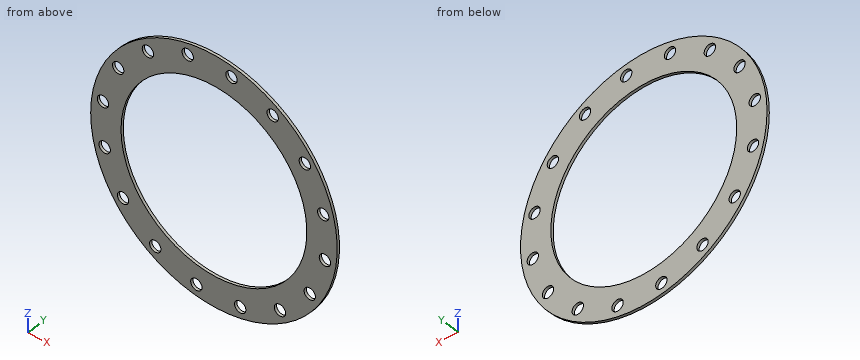
Autodesk Inventor part; units mm, degrees
ref_plane "YZ Plane" through (0, 0, 0) normal (1, 0, 0) x (0, 1, 0)
ref_plane "XZ Plane" through (0, 0, 0) normal (0, 1, 0) x (-1, 0, 0)
ref_plane "XY Plane" through (0, 0, 0) normal (0, 0, 1) x (1, 0, 0)
sketch "Sketch1" plane through (0, 0, 0) normal (0, 1, 0) x (-1, 0, 0)
  circle A0 centre (0, 0) radius 213
  circle A1 centre (0, 0) radius 282.5
  line L0 (282.5, 0) -> (213, 0)
  line L1 (-213, 0) -> (-282.5, 0)
  line L2 (0, 213) -> (0, 282.5)
  point P0 (247.75, 0)
  point P1 (-247.75, 0)
  point P2 (0, 247.75)
  dimension "d1" = 565
  dimension "d4" = 426
extrude "Extrusion1" add sketch "Sketch1" along normal blind 6 contours L0 A1 L1 A0 | A0 L2 A1 L0 | A0 L1 A1 L2
sketch "Sketch2" plane through (0, 0, 0) normal (0, -1, 0) x (1, 0, 0)
  circle A0 centre (0, 0) radius 282.5
  circle A1 centre (0, 0) radius 213
  circle A2 centre (40.2819, 254.3297) radius 13
  circle A3 centre (0, 0) radius 213
  line L0 (40.2819, 254.3297) -> (0, 0)
  point P0 (0, 213)
  point P1 (265, 0)
  dimension "d5" = 257.5
  dimension "d7" = 26
extrude "Cut1" cut sketch "Sketch2" against normal blind 6 contours A2
pattern_circular "Circular Pattern1" count 16 over 360 about axis through (0, 0, 0) along (0, 1, 0) of "Cut1"
equation "\"d1\" = Charging_hatch_width"
equation "\"d4\" = Accsess_hatch_diameter"
equation "\"d9\" = Thickness"
equation "\"BendRadius\" = Thickness"
equation "\"BendReliefWidth\" = Thickness"
equation "\"BendReliefDepth\" = 0.5 * Thickness"
equation "\"CornerReliefSize\" = 4 * Thickness"
equation "\"MinimumRemnant\" = 2 * Thickness"
equation "\"TransitionRadius\" = BendRadius"
equation "\"JacobiRadiusSize\" = BendRadius"
equation "\"GapSize\" = Thickness"
equation "\"d8\" = Thickness"
properties part number "TZS 1203 accses hatch flange" material "Steel"
Build history of the part. All positions in model axes, mm. Round coordinates to 2 decimals unless told otherwise and drop trailing zeros. Loops run counter-clockwise (first coordinate to the right, second up) from the corner with the lowest first, then second, coordinate; pieces in that order, holes last. Notation, with made-up numbers: M 58,53.5 L 75,53.5 A19 cw 75,89.5 Z; hole C 1,82 d10. An arc over 180 degrees is marked long. Answer as CSV lines item,"result".
1. Cut at A-A on x = 0. Write the cut outline in (y, z).
Resolved:
outline,"M 0,-282.5 L 6,-282.5 L 6,-213 L 0,-213 Z; M 0,213 L 6,213 L 6,282.5 L 0,282.5 Z"
2. Flat gauge pins, fed straight in: P1, Ø1.5, axis at y = 1, z = 131.5, coming from the -X side; P2, Ø6, axis at x = 52, z = 213.5, coming from the -Y side; P3, Ø3, axis at x = 192, y = 0.5, coming from the -Z side; P4, Ø3, axis at x = 223, y = 2.5, coming from the -Z side. Where does each tip first touch, or does it go through?
Resolved:
P1,"stops at x = -250.42"
P2,"stops at y = 0"
P3,"stops at z = -208.6"
P4,"stops at z = -175.34"
3. Wall check: probe 1 along X at (y, z) = (4.15, 150.5); probe 2 along X at (y, z) = (4.6, -256.5); probe 3 along Z at (x, y) = (-146, 3.45). Give the ranges that are in metal, low to high. Write a range as [from, to].
Resolved:
probe 1,"x = [-239.07, -150.73], [150.73, 195.35], [221.29, 239.07]"
probe 2,"x = [-118.38, -53.1], [-27.46, 48.64], [71.58, 118.38]"
probe 3,"z = [-241.85, -225.7], [-213.41, -155.09], [155.09, 196.48], [220.17, 241.85]"
4. Cut at B-B on z = 0. Write the cut outline in (x, y).
Resolved:
outline,"M -282.5,0 L -213,0 L -213,6 L -282.5,6 Z; M 213,0 L 282.5,0 L 282.5,6 L 213,6 Z"
